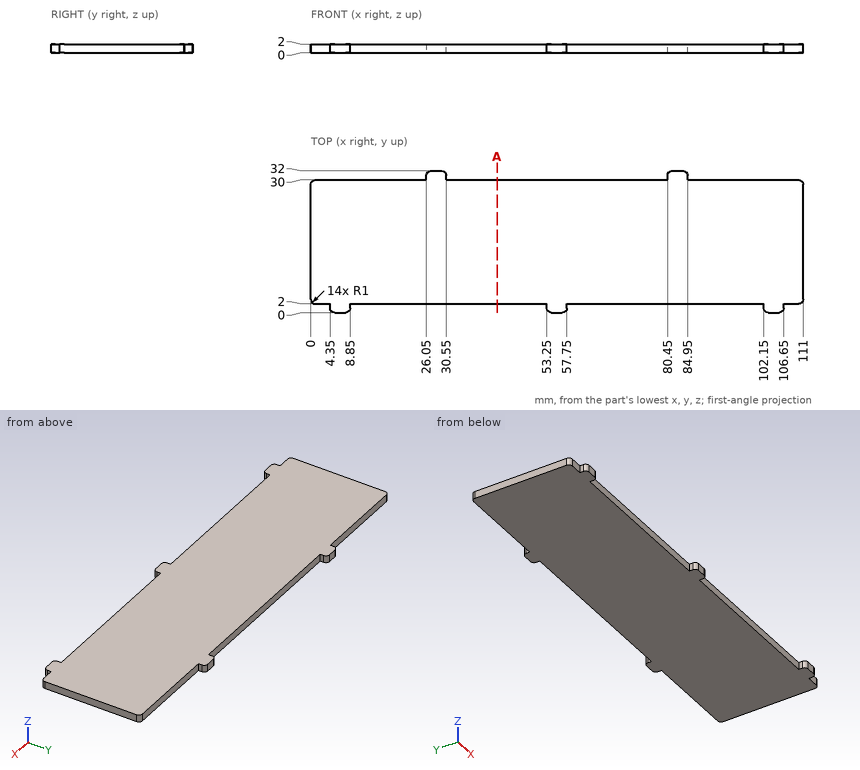
For this review, use the dimensioned drawing (mm, ordinates from the lowest corner) and the shaded views. Round coordinates to 2 decimals unless told otherwise and drop trailing zeros. Order: outer loops, then holes, each group sorted by start corner. A loop starts at its lowest first (then second) coordinate and runs counter-clockwise, first axis right, second up. Notation, with made-up numbers: M -14,-28.75 L 7,-28.75 A15 ccw 7,-0.75 Z; hole C 64,-23 d5. An arc over 180 degrees is marked long. Use a Markdown table: item, result. Add a question column.
Item 1: Insertion check: pin 1 (0.8 mm diameter, centred on y = 1.5, z = 1, fed in from +X); pin 2 (1 mm diameter, centred on x = 42.5, z = 1, fed in from -Y); pin 3 (0.5 mm diameter, centred on y = 30.5, z = 0.5, fed in from -X). Each pin has a flat end and moves straight along its axis. Give the tip position at first contact, or say it passes through.
Item 2: To check wall thickness, follow line 1 along X through (y, z) = (30.5, 1.3); line 2 along Y through (x, z) = (33.5, 0.85); line 3 along Y through (x, z) = (27, 1.1). State the ranges of each line that lie inside material, in increasing order.
Item 3: Add section A-A, the plane x = 42. Give the boundary of the cut face in (y, z).
Geometry results:
| question | item | result |
|---|---|---|
| 1 | pin 1 | stops at x = 106.65 |
| 1 | pin 2 | stops at y = 2 |
| 1 | pin 3 | stops at x = 26.05 |
| 2 | line 1 | x = 26.05 to 30.55, 80.45 to 84.95 |
| 2 | line 2 | y = 2 to 30 |
| 2 | line 3 | y = 2 to 32 |
| 3 | outline | M 2,0 L 30,0 L 30,2 L 2,2 Z |
